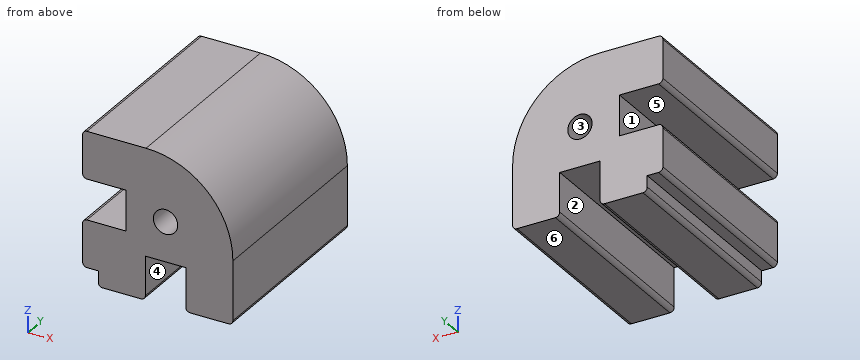
from build123d import *

# Parameters (mm, degrees)
SKETCH1_R           = 2.8
BOSS_EXTRUDE1_DEPTH = 45
FILLET1_R           = 1
FILLET2_R           = 20


with BuildPart() as part:
    # Sketch1 → Boss-Extrude1 (new body)
    with BuildSketch(Plane(origin=(0, 0, 0), x_dir=(1, 0, 0), z_dir=(0, 1, 0))):
        Polygon((-19.099152542, -15.5), (-19.099152542, -4.65), (-9.099152542, -4.65), (-9.099152542, 4.65), (-19.099152542, 4.65), (-19.099152542, 15.5), (-15.5, 15.5), (-15.5, 19.099152542), (-4.65, 19.099152542), (-4.65, 9.099152542), (4.65, 9.099152542), (4.65, 19.099152542), (15.5, 19.099152542), (15.5, -15.5), align=None)
        with Locations(Location((0, 0, 0), (0, 0, 90))):
            Circle(SKETCH1_R, mode=Mode.SUBTRACT)
    extrude(amount=BOSS_EXTRUDE1_DEPTH)

    # Fillet1
    fillet1_edges = [part.edges().sort_by_distance(p)[0] for p in [
        (-19.099152542, 22.5, 15.5),
        (-19.099152542, 22.5, 4.65),
        (-19.099152542, 22.5, -4.65),
        (-19.099152542, 22.5, -15.5),
        (-15.5, 22.5, -19.099152542),
        (-4.65, 22.5, -19.099152542),
        (4.65, 22.5, -19.099152542),
        (15.5, 22.5, -19.099152542),
    ]]
    fillet(fillet1_edges, radius=FILLET1_R)

    # Fillet2
    fillet2_edges = [part.edges().sort_by_distance(p)[0] for p in [
        (15.5, 22.5, 15.5),
    ]]
    fillet(fillet2_edges, radius=FILLET2_R)


solid = part.part
Build history of the part. All positions in model axes, mm. Face numbers are marked on the shaded views. A direction names the side the tool comes from. Round coordinates to 2 decimals unless told otherwise and drop trailing zeros. Write each loop counter-clockwise with the first axis right and the second up, starting at its lowest first coordinate (ties: lowest second). Pieces come first, ordered by that corner, then holes. Notation, with made-up numbers: M 2,-9.5 L 27,-9.5 A6 cw 27,-0.5 Z; hole C 87.5,27.5 d10. An arc over 180 degrees is marked long. Answer as a JSON object with one key per item and string values. Group by question number.
(1) Drill centre lines: L1, parallel to X at y = 8, z = -13; L2, parallel to Z at x = -17, y = 7. Where is each one in solid material? Low to high.
(2) Cut at A-A (x = -12.5). Give the cut face in (y, z).
(3) Mould opens along Z. For the marked faces 4, 5 and 6 say: pulls with the +Z half, pulls with the -Z half, needs draft (parallel to the pull), parting line crosses it, or undercut.
(4) Cut at B-B (y = 25). Give the cut face in (x, z).
(5) Flat gauge pins, fed straight in: pin 1 (7.5 mm diameter, centred on x = 0, z = 0, fed in from +Y); pin 2 (6 mm diameter, centred on y = 16.5, z = 5.5, fed in from +X) (3 decimals); pin 3 (0.8 mm diameter, centred on x = -17, y = 12, fed in from -Z); pin 4 (7.5 mm diameter, centred on x = 1.5, y = 17, fed in from -Z). Where does each tip first touch, or does it go through?
(6) Which spindle directions (+Z, -Z, +X, -X, +Y, -Y) get a long thin tool onto all of the face, cutting with end or side? Do the marked faces 1, 2 and 3. Say none if no direction does.
(7) Cut at C-C (z = 0). Give the cut face in (x, y), and give its area (3 significant figures).
(8) Cut at D-D (x = 11.5). Give the cut face in (y, z), and give its area (3 significant figures).
Responses:
{
 "1": {"L1": "x = -19.1 to -4.65, 4.65 to 15.5", "L2": "z = -15.5 to -4.65, 4.65 to 15.5"},
 "2": {"outline": "M 0,-19.1 L 45,-19.1 L 45,-4.65 L 0,-4.65 Z; M 0,4.65 L 45,4.65 L 45,15.5 L 0,15.5 Z"},
 "3": {"face 4": "needs draft", "face 5": "undercut", "face 6": "pulls with the -Z half"},
 "4": {"outline": "M -19.1,-14.5 A1 ccw -18.1,-15.5 L -15.5,-15.5 L -15.5,-18.1 A1 ccw -14.5,-19.1 L -5.65,-19.1 A1 ccw -4.65,-18.1 L -4.65,-9.1 L 4.65,-9.1 L 4.65,-18.1 A1 ccw 5.65,-19.1 L 14.5,-19.1 A1 ccw 15.5,-18.1 L 15.5,-4.5 A20 ccw -4.5,15.5 L -18.1,15.5 A1 ccw -19.1,14.5 L -19.1,5.65 A1 ccw -18.1,4.65 L -9.1,4.65 L -9.1,-4.65 L -18.1,-4.65 A1 ccw -19.1,-5.65 Z; hole C 0,0 d5.6"},
 "5": {"pin 1": "stops at y = 45", "pin 2": "stops at x = 14.235", "pin 3": "stops at z = -15.5", "pin 4": "stops at z = -19.02"},
 "6": {"face 1": "-X, +Y, -Y", "face 2": "-Z, +Y, -Y", "face 3": "+Y, -Y"},
 "7": {"outline": "M -9.1,0 L -2.8,0 L -2.8,45 L -9.1,45 Z; M 2.8,0 L 14.99,0 L 14.99,45 L 2.8,45 Z", "area": "832 mm2"},
 "8": {"outline": "M 0,-19.1 L 45,-19.1 L 45,7.5 L 0,7.5 Z", "area": "1,200 mm2"}
}
